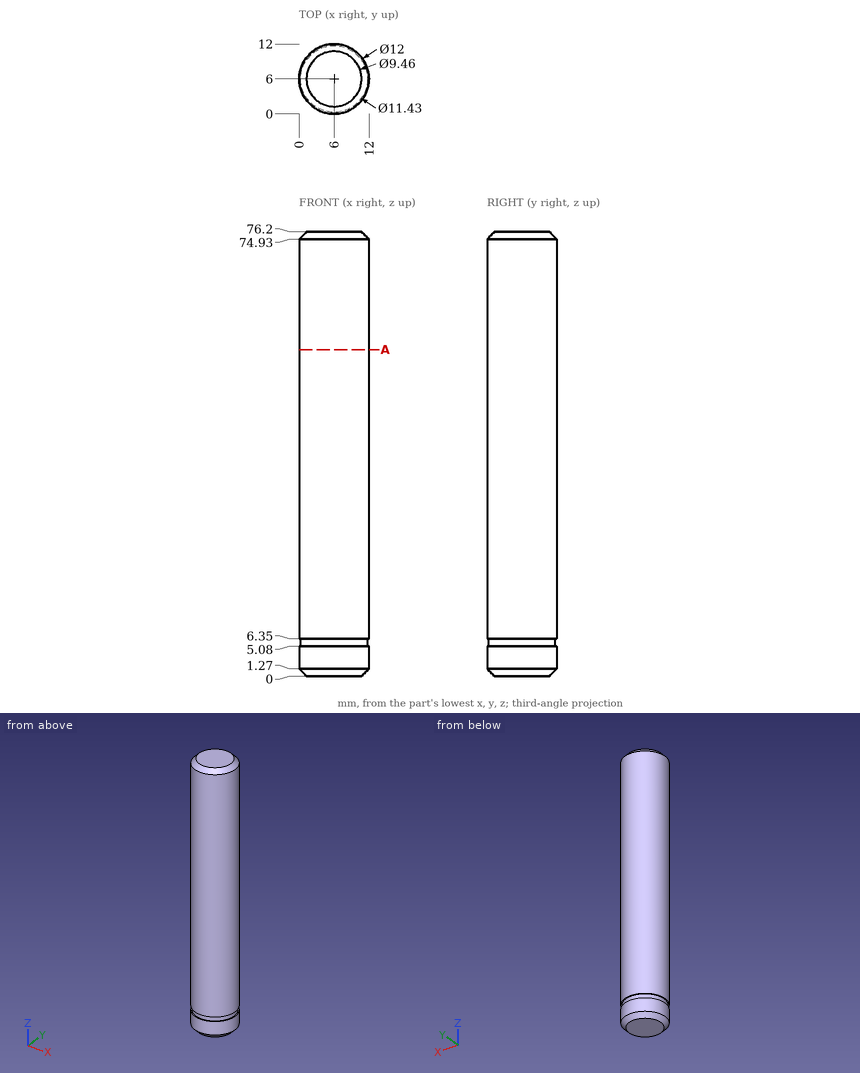
Source: three-view drawing plus pictorial views. Frame: mm from the lowest corner of the part. Round coordinates to 2 decimals unless told otherwise and drop trailing zeros. Order: outer loops, then holes, each group sorted by start corner. A loop starts at its lowest first (then second) coordinate and runs counter-clockwise, first axis right, second up. Notation, with made-up numbers: (62.5, -4.75) -> (82.5, -4.75) arc R9 cw to (82.5, 12.25) -> close; hole circle Ø5 at (56, -33.5). An arc over 180 degrees is marked (long way). Use CSV: the item, a comma, the result in double quotes. Start each with the question number.
1) Section A-A (z = 56). Return the cut outline in (x, y).
2) Material intervals for line 1 along Y through (x, z) = (6.25, 73); line 2 along X through (y, z) = (3.5, 42.5); line 3 along Z through (x, y) = (1.5, 8.5), sorted ascending. Write a range as from..to.
3) First-contact query: pin 1 Ø6 at (y, z) = (1.5, 23.5) entering from +X; pin 2 Ø4 at (x, z) = (6.5, 50.5) entering from +Y; pin 3 Ø6 at (x, z) = (9.5, 16) entering from -Y; pin 4 Ø2 at (y, z) = (2, 36.5) entering from +X. Flat tips, straight axial feed; report the tip coordinate or a pass-through.
Returned:
1,outline,"circle Ø12 at (6, 6)"
2,line 1,"y = 0.01..11.99"
2,line 2,"x = 0.55..11.45"
2,line 3,"z = 0.42..75.78"
3,pin 1,"stops at x = 11.81"
3,pin 2,"stops at y = 12"
3,pin 3,"stops at y = 0.02"
3,pin 4,"stops at x = 11.2"
